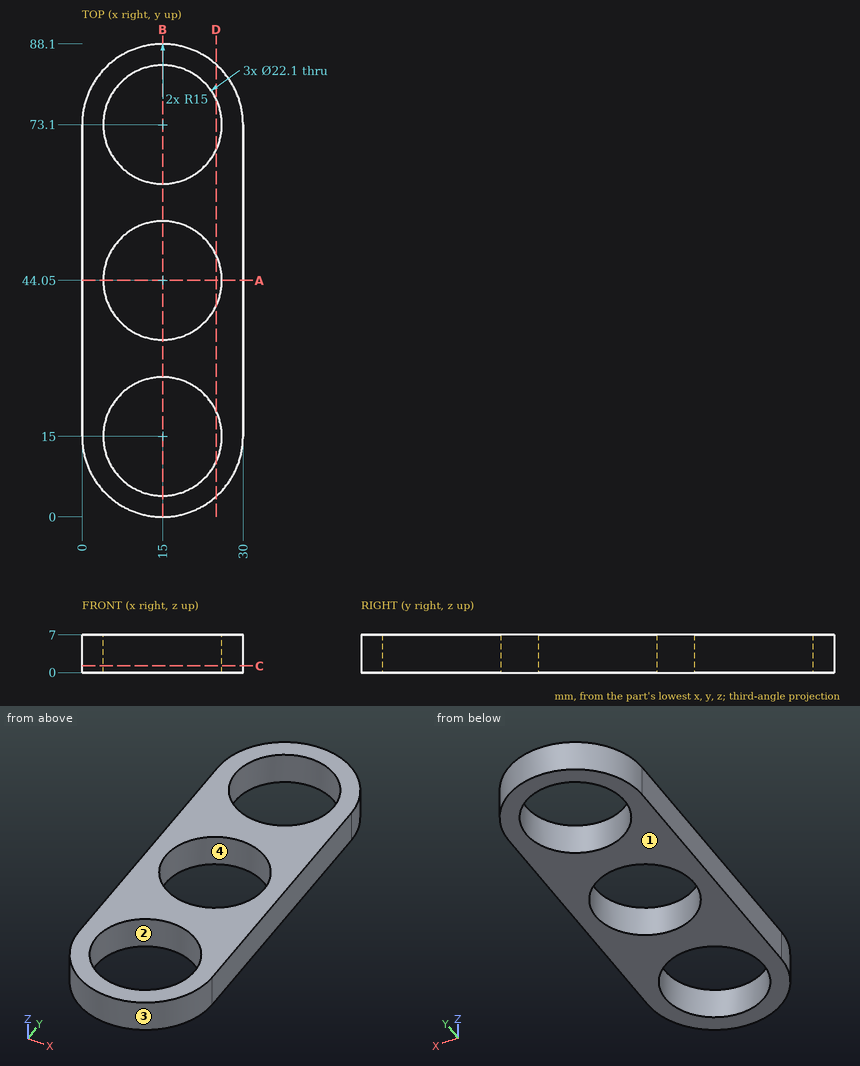
Verification items for this drawing (mm, ordinates from the low corner). Give positions to 0.01 mm unless a question says otherwise; leave off trailing zeros. Loops run counter-clockwise (first coordinate to the right, second up) from the corner with the lowest first, then second, coordinate; pieces in that order, holes last. Notation, with made-up numbers: M 82.5,43 L 124.5,43 A20 ccw 124.5,61 Z; hole C -16,-7 d1. An arc over 180 degrees is marked long. Answer as a JSON object with one key per item and string values. Group by question number.
Q1. Release check for a two-part mould opening along X. For the marked faces 1, 2, 3 and 4 record: released by +X, released by -X, zero draft, split by the parting line, or undercut.
Q2. Cross-section at B-B on x = 15. Record the cut outline in (y, z), then the cut area to 3 significant figures.
Q3. Material ranges on line 1 along Y through (x, z) = (15, 2.25); line 2 along X through (y, z) = (72.5, 1.25); line 3 along Y through (x, z) = (8.5, 4.75), recorded low to high. Write a range as [from, to].
Q4. Cross-section at A-A on y = 44.05. Record the cut outline in (x, z).
Q5. Go/stop test with flat-tipped pins: P1, Ø1.5, axis at x = 3.5, y = 25, coming from the -Z side; P2, Ø3, axis at x = 20, z = 6, coming from the +Y side; P3, Ø2, axis at x = 27, z = 5, coming from the +Y side; P4, Ø1, axis at x = 23, z = 3.5, coming from the -Y side. Record where each tip stops, or that it passes through.
Q6. Cross-section at C-C on z = 1.25. Record the cut outline in (x, y).
Q7. Cross-section at D-D on x = 25. Record the cut outline in (y, z), then the cut area to 3 significant figures.
Evaluation:
{
 "1": {"face 1": "zero draft", "face 2": "undercut", "face 3": "split by the parting line", "face 4": "undercut"},
 "2": {"outline": "M 0,0 L 3.95,0 L 3.95,7 L 0,7 Z; M 26.05,0 L 33,0 L 33,7 L 26.05,7 Z; M 55.1,0 L 62.05,0 L 62.05,7 L 55.1,7 Z; M 84.15,0 L 88.1,0 L 88.1,7 L 84.15,7 Z", "area": "153 mm2"},
 "3": {"line 1": "y = [0, 3.95], [26.05, 33], [55.1, 62.05], [84.15, 88.1]", "line 2": "x = [0, 3.97], [26.03, 30]", "line 3": "y = [1.48, 6.06], [23.94, 35.11], [52.99, 64.16], [82.04, 86.62]"},
 "4": {"outline": "M 0,0 L 3.95,0 L 3.95,7 L 0,7 Z; M 26.05,0 L 30,0 L 30,7 L 26.05,7 Z"},
 "5": {"P1": "stops at z = 0", "P2": "stops at y = 87.69", "P3": "stops at y = 83.3", "P4": "stops at y = 2.01"},
 "6": {"outline": "M 0,15 A15 ccw 30,15 L 30,73.1 A15 ccw 0,73.1 Z; hole C 15,15 d22.1; hole C 15,44.05 d22.1; hole C 15,73.1 d22.1"},
 "7": {"outline": "M 3.82,0 L 10.3,0 L 10.3,7 L 3.82,7 Z; M 19.7,0 L 39.35,0 L 39.35,7 L 19.7,7 Z; M 48.75,0 L 68.4,0 L 68.4,7 L 48.75,7 Z; M 77.8,0 L 84.28,0 L 84.28,7 L 77.8,7 Z", "area": "366 mm2"}
}
